```python
from build123d import *

# Parameters (mm, degrees)
BOSS_EXTRUDE1_DEPTH = 1.4
FILLET1_R           = 2


with BuildPart() as part:
    # Sketch2 → Boss-Extrude1 (new body, symmetric)
    with BuildSketch(Plane.XY):
        Polygon((-23.168593437, 25), (-12.682504049, 14.513910612), (-14.513910612, 12.682504049), (-25, 23.168593437), (-25, 1.325866762), (-19.261635993, 1.325866762), (-19.261635993, -1.264133238), (-25, -1.264133238), (-25.074518955, -23.137726675), (-14.588429567, -12.651637287), (-12.757023004, -14.48304385), (-23.243112392, -24.969133238), (-1.400385717, -25), (-1.400385717, -19.230769231), (1.189614283, -19.230769231), (1.189614283, -25), (23.063207719, -25.043652193), (12.577118332, -14.557562806), (14.408524895, -12.726156242), (24.894614283, -23.21224563), (25, -1.369518955), (19.156250275, -1.369518955), (19.156250275, 1.220481045), (25, 1.220481045), (24.969133238, 23.094074481), (14.48304385, 12.607985094), (12.651637287, 14.439391657), (23.137726675, 24.925481045), (1.295, 25), (1.295, 19.187117037), (-1.295, 19.187117037), (-1.295, 25), align=None)
    extrude(amount=BOSS_EXTRUDE1_DEPTH, both=True)

    # Fillet1
    fillet1_edges = [part.edges().sort_by_distance(p)[0] for p in [
        (-1.295, 25, 0),
        (1.295, 25, 0),
        (23.137726675, 24.925481045, 0),
        (24.969133238, 23.094074481, 0),
        (25, 1.220481045, 0),
        (25, -1.369518955, 0),
        (24.894614283, -23.21224563, 0),
        (23.063207719, -25.043652193, 0),
        (1.189614283, -25, 0),
        (-1.400385717, -25, 0),
        (-23.243112392, -24.969133238, 0),
        (-25.074518955, -23.137726675, 0),
        (-25, -1.264133238, 0),
        (-25, 1.325866762, 0),
        (-25, 23.168593437, 0),
        (-23.168593437, 25, 0),
    ]]
    fillet(fillet1_edges, radius=FILLET1_R)


solid = part.part
```
Input: part model. Units: mm. Frame: model coordinates. A direction names the side the tool comes from. Round coordinates to 2 decimals unless told otherwise and drop trailing zeros. Loops run counter-clockwise (first coordinate to the right, second up) from the corner with the lowest first, then second, coordinate; pieces in that order, holes last. Notation, with made-up numbers: (85, -8.5) -> (117, -8.5) arc R17 ccw to (117, 5.5) -> close; hole circle Ø9 at (-34.75, 66). An arc over 180 degrees is marked (long way). Write each question's results on one line, items separated by ' | '.
1. Ray query, line 1 (Y direction, x = 15.5, z = 0.4); line 2 (Y direction, x = -15.5, z = -0.05); line 3 (X direction, y = 14, z = -0.2). Return the intervals inside material, ascending. Write a range as from..to.
Geometry results:
line 1: -25.03..-17.48, -13.82..13.62, 17.29..24.95 | line 2: -24.98..-17.23, -13.56..13.67, 17.33..25 | line 3: -25..-15.83, -13.2..13.09, 15.88..24.98
2. Mould query, pull axis X, two halves, no side actions, for faces 1 (the face through (-16.247, -17.973, 0.02)), 2 (the face through (-21, 1.326, 0)), 3 (the face through (-25, 11, 0)). Classes: +X half, -X half, draft (parallel to the pull), parting line (faces both ways), or undercut.
Geometry results:
face 1: undercut | face 2: draft | face 3: -X half
3. Section B-B (y = -0.5). Return loops of the section in (x, z).
Geometry results:
outline: (-19.26, -1.4) -> (19.16, -1.4) -> (19.16, 1.4) -> (-19.26, 1.4) -> close
4. Section A-A (y = 15.5). Return loops of the section in (x, z), and give its area (3 significant figures).
Geometry results:
outline: (-25, -1.4) -> (-17.33, -1.4) -> (-17.33, 1.4) -> (-25, 1.4) -> close; (-13.67, -1.4) -> (13.71, -1.4) -> (13.71, 1.4) -> (-13.67, 1.4) -> close; (17.38, -1.4) -> (24.98, -1.4) -> (24.98, 1.4) -> (17.38, 1.4) -> close | area: 119 mm2
5. First-contact query: P1, Ø1.4, axis at y = 20.5, z = 0, coming from the -X side; P2, Ø0.8, axis at x = -20.5, z = 0, coming from the +Y side; P3, Ø0.8, axis at x = -0.5, z = -0.5, coming from the +Y side. Flat tips, straight axial feed; report the tip coordinate or a pass-through.
Geometry results:
P1: x = -24.37 | P2: y = 23.95 | P3: y = 19.19
6. Set-up query: faces 4 (the face through (23.709, -20.244, 0.02)), 5 (the face through (-24.4, 1.9, 0)), 6 (the face through (18.072, 16.197, 0.02)), 7 (the face through (21, -1.37, 0)), 8 (the face through (-1.295, 21, 0)). Return all of +Z, -Z, +X, -X, +Y, -Y with unobstructed straight access to the full face (end or side cutting, diameter ignored); none if empty.
Geometry results:
face 4: +Z, -Z, -Y | face 5: +Z, -Z, -X | face 6: +Z, -Z | face 7: +Z, -Z, +X | face 8: +Z, -Z, +Y
